Autodesk Inventor part; units mm, degrees
ref_plane "YZ Plane" through (0, 0, 0) normal (1, 0, 0) x (0, 1, 0)
ref_plane "XZ Plane" through (0, 0, 0) normal (0, 1, 0) x (-1, 0, 0)
ref_plane "XY Plane" through (0, 0, 0) normal (0, 0, 1) x (1, 0, 0)
sketch "Sketch1" plane through (0, 0, 0) normal (1, 0, 0) x (0, 1, 0)
  line L0 (0, 0) -> (0, -9)
  line L1 (0, -9) -> (-1, -9)
  line L2 (-1, -9) -> (-1, -13)
  line L3 (-1, -13) -> (-3.5, -13)
  line L4 (-3.5, -13) -> (-3.5, -22)
  line L5 (-3.5, -22) -> (-4, -22)
  line L6 (-4, -22) -> (-4, -34)
  line L7 (-4, -34) -> (-5.1, -36)
  line L8 (-5.1, -36) -> (-6, -36)
  line L9 (0, 0) -> (-2.2, -2.5)
  line L10 (-2.2, -2.5) -> (-2.2, -9)
  line L11 (-6, -9.5) -> (-6, -36)
  line L12 (-2.2, -9) -> (-6, -9.5)
  dimension "d0" = 9
  dimension "d1" = 4
  dimension "d2" = 1
  dimension "d3" = 2.5
  dimension "d4" = 9
  dimension "d5" = 12
  dimension "d6" = 2
  dimension "d7" = 2
  dimension "d9" = 2.2
  dimension "d10" = 2.5
  dimension "d11" = 6.5
  dimension "d12" = 0.5
  dimension "d14" = 0.5
  dimension "d15" = 1.1
revolve "Revolution1" add sketch "Sketch1" angle 360 about axis through (0, -6, -9.5) along (0, 0, -1)
sketch "Sketch3" plane through (0, 0, 0) normal (1, 0, 0) x (0, 1, 0)
  line L0 (-4.75, 0) -> (-7.25, 0)
  line L1 (-7.25, 0) -> (-7.25, -10)
  line L2 (-4.75, -10) -> (-4.75, 0)
  arc A0 (-7.25, -10) -> (-4.75, -10) centre (-6, -10) ccw
  line L3 (0, -43.2) -> (0, 7.2)
  line L4 (-14.4, 0) -> (2.4, 0)
  point P0 (0, 0)
  dimension "d19" = 2.5
  dimension "d20" = 10
  dimension "d21" = 6
extrude "Extrusion1" cut sketch "Sketch3" along normal through all both and the other way through all
sketch "Sketch4" plane through (0, 0, 0) normal (1, 0, 0) x (0, 1, 0)
  circle A0 centre (-6, -20) radius 1.1
  line L0 (0, -43.2) -> (0, 7.2)
  line L1 (-14.4, 0) -> (2.4, 0)
  point P0 (0, 0)
  dimension "d24" = 2.2
  dimension "d25" = 6
  dimension "d26" = 20
extrude "Extrusion2" cut sketch "Sketch4" along normal through all both and the other way through all
thread "Thread1"
properties part number "RCT-H005"
For this review, take the finished solid that the model builds, in its own axes (mm). A direction names the side the tool comes from. Round coordinates to 2 decimals unless told otherwise and drop trailing zeros. Write each loop counter-clockwise with the first axis right and the second up, starting at its lowest first coordinate (ties: lowest second). Pieces come first, ordered by that corner, then holes. Notation, with made-up numbers: (-30, -32.5) -> (-1, -32.5) arc R34 ccw to (-1, 3.5) -> close; hole circle Ø7 at (73.5, 46.25). An arc over 180 degrees is marked (long way). One line per question, with ' | ' between items. Start each with the question number.
1) Wall thickness on line 1 along Z through (x, y) = (0.8, -6); line 2 along Y through (x, z) = (0.1, -20); line 3 along Y through (x, z) = (-1.5, -14.5): over which ranges is each line inside the solid? List them lowest first.
2) Add section B-B (x = 0). Write out the cut boundary in (y, z), and give its area (3 significant figures).
3) Mouldability with a two-part tool opening along Z and no side actions: class faces 1 (the flat face through (0, -6, -36)), 2 (the cylindrical face through (0.035, -4.984, -20.421)), 3 (the cylindrical face through (-0.07, -5.97, -11.25)) as +Z half, -Z half, draft (parallel to the pull), parting line (faces both ways), or undercut.
4) Machinability: for faces 4 (the flat face through (-0.1, -4.75, -9.5)), 5 (the cylindrical face through (-1.2, -7.6, -28.1)), 6 (the conical face through (0.039, -3.741, -9.203)), which of the approach directions +Z, -Z, +X, -X, +Y, -Y give a long, thin tool a straight path to every point of the face, cutting with its end or side? Answer none if there is none.
5) Add section A-A (y = -6). Write out the cut boundary in (x, z), and give its area (3 significant figures).
6) For pin 1 Ø1.4 at (x, y) = (0.5, -2.5) entering from -Z; pin 2 Ø6 at (y, z) = (-10, -19.5) entering from +X; pin 3 Ø6 at (x, z) = (-4.5, -17) entering from +Y, all flat-tipped, find the tip position at first contact; note any pin that passes through.
7) Add section C-C (z = -18). Write out the cut boundary in (x, y).
8) Add section D-D (z = -22.5). Write out the cut boundary in (x, y), and give its area (3 significant figures).
Reported:
1) line 1: z = -36 to -21.1, -18.9 to -11.25 | line 2: y = -8.5 to -7.1, -4.9 to -3.5 | line 3: y = -8 to -4
2) outline: (-12, -9) -> (-11, -9) -> (-11, -13) -> (-8.5, -13) -> (-8.5, -22) -> (-8, -22) -> (-8, -34) -> (-6.9, -36) -> (-5.1, -36) -> (-4, -34) -> (-4, -22) -> (-3.5, -22) -> (-3.5, -13) -> (-1, -13) -> (-1, -9) -> (0, -9) -> (0, 0) -> (-2.2, -2.5) -> (-2.2, -9) -> (-4.75, -9.34) -> (-4.75, -10) arc R1.25 cw to (-7.25, -10) -> (-7.25, -9.34) -> (-9.8, -9) -> (-9.8, -2.5) -> (-12, 0) -> close; hole circle Ø2.2 at (-6, -20) | area: 163 mm²
3) face 1: -Z half | face 2: undercut | face 3: +Z half
4) face 4: +Z, +X, -X | face 5: -Z | face 6: +Z
5) outline: (-5, -13) -> (-2.5, -13) -> (-2.5, -18.9) -> (2.5, -18.9) -> (2.5, -13) -> (5, -13) -> (5, -11.25) -> (-5, -11.25) -> close; (-2.5, -22) -> (-2, -22) -> (-2, -34) -> (-0.9, -36) -> (0.9, -36) -> (2, -34) -> (2, -22) -> (2.5, -22) -> (2.5, -21.1) -> (-2.5, -21.1) -> close | area: 105 mm²
6) pin 1: stops at z = -13 | pin 2: stops at x = 2.29 | pin 3: stops at y = -4
7) outline: circle Ø5 at (0, -6)
8) outline: circle Ø4 at (0, -6) | area: 12.6 mm²
